from build123d import *

# Parameters (mm, degrees)
SKETCH_3_W          = 11
SKETCH_3_H          = 20
SKETCH_3_R          = 1.6
SKETCH_3_R_2        = 1.225
EXTRUDE_1_DEPTH     = 21.25
SKETCH_4_W          = 3
SKETCH_4_H          = 5.7
CUT_EXTRUDE_1_DEPTH = 7.1


with BuildPart() as part:
    # 草图3 → 凸台-拉伸1 (new body)
    with BuildSketch(Plane.XY):
        with Locations((5.5, 10)):
            Rectangle(SKETCH_3_W, SKETCH_3_H)
        with Locations((3.5, 14.85)):
            Circle(SKETCH_3_R, mode=Mode.SUBTRACT)
        with Locations((3.5, 5.15)):
            Circle(SKETCH_3_R, mode=Mode.SUBTRACT)
        with Locations((8.15, 14.85)):
            Circle(SKETCH_3_R_2, mode=Mode.SUBTRACT)
        with Locations((8.15, 5.15)):
            Circle(SKETCH_3_R_2, mode=Mode.SUBTRACT)
    extrude(amount=EXTRUDE_1_DEPTH)

    # 草图4 → 切除-拉伸1 (cut)
    with BuildSketch(Plane.ZY):
        with Locations((4.5, 14.85)):
            Rectangle(SKETCH_4_W, SKETCH_4_H)
        with Locations((4.5, 5.15)):
            Rectangle(SKETCH_4_W, SKETCH_4_H)
    extrude(amount=-CUT_EXTRUDE_1_DEPTH, mode=Mode.SUBTRACT)


solid = part.part
The model under review builds one solid part; all positions refer to its coordinate system, in mm. A direction names the side the tool comes from. Round coordinates to 2 decimals unless told otherwise and drop trailing zeros. Write each loop counter-clockwise with the first axis right and the second up, starting at its lowest first coordinate (ties: lowest second). Pieces come first, ordered by that corner, then holes. Notation, with made-up numbers: M 79,0.5 L 103,0.5 A11 cw 103,5.5 Z; hole C 12,63 d6. An arc over 180 degrees is marked long. Use a Markdown table: item, result. Add a question column.
Q1. We need section B-B, the plane y = 5.15. State the section outline as (x, z) points (3 decimals), plus the area to 3 significant figures.
Q2. To check wall thickness, follow line 1 (X direction, y = 14.85, z = 18.25) (3 decimals); line 2 (Y direction, x = 3.5, z = 18); line 3 (Y direction, x = 8.25, z = 3.25). State the ranges of each line that lie inside material, in increasing order.
Q3. Insertion check: pin 1 (2.5 mm diameter, centred on x = 3.5, y = 5.15, fed in from +Z); pin 2 (1.1 mm diameter, centred on y = 3.5, z = 5, fed in from -X). Each pin has a flat end and moves straight along its axis. Give the tip position at first contact, or say it passes through.
Q4. Machinability: for faces 4 (the face through (3.292, 6.736, 1.479)), 5 (the face through (4, 17.7, 4)), which of the approach directions +Z, -Z, +X, -X, +Y, -Y give a long, thin tool a straight path to every point of the face, cutting with its end or side? Answer none if there is none.
Q5. We need section A-A, the plane x = 3.5. State the section outline as (y, z) points.
Q6. We need section D-D, the plane z = 13.5. State the section outline as (x, y) points (3 decimals).
Q7. The part is to be moulded in two halves that separate along Y. For faces 1 (the face through (4, 12, 4)), 2 (the face through (5, 0, 10)), 3 (the face through (11, 10, 10)), say which applies: pulls with the +Y half, pulls with the -Y half, needs draft (parallel to the pull), parting line crosses it, or undercut.
Q8. We need section C-C, the plane x = 6. State the section outline as (y, z) points, plus the area to 3 significant figures.
Findings below:
| question | item | result |
|---|---|---|
| 1 | outline | M 0,0 L 1.9,0 L 1.9,3 L 0,3 Z; M 0,6 L 1.9,6 L 1.9,21.25 L 0,21.25 Z; M 5.1,0 L 6.925,0 L 6.925,3 L 5.1,3 Z; M 5.1,6 L 6.925,6 L 6.925,21.25 L 5.1,21.25 Z; M 9.375,0 L 11,0 L 11,21.25 L 9.375,21.25 Z |
| 1 | area | 103 mm² |
| 2 | line 1 | x = 0 to 1.9, 5.1 to 6.925, 9.375 to 11 |
| 2 | line 2 | y = 0 to 3.55, 6.75 to 13.25, 16.45 to 20 |
| 2 | line 3 | y = 0 to 3.93, 6.37 to 13.63, 16.07 to 20 |
| 3 | pin 1 | passes through |
| 3 | pin 2 | stops at x = 7.1 |
| 4 | face 4 | +Z, -Z |
| 4 | face 5 | -X |
| 5 | outline | M 0,0 L 3.55,0 L 3.55,3 L 2.3,3 L 2.3,6 L 3.55,6 L 3.55,21.25 L 0,21.25 Z; M 6.75,0 L 13.25,0 L 13.25,3 L 12,3 L 12,6 L 13.25,6 L 13.25,21.25 L 6.75,21.25 L 6.75,6 L 8,6 L 8,3 L 6.75,3 Z; M 16.45,0 L 20,0 L 20,21.25 L 16.45,21.25 L 16.45,6 L 17.7,6 L 17.7,3 L 16.45,3 Z |
| 6 | outline | M 0,0 L 11,0 L 11,20 L 0,20 Z; hole C 3.5,5.15 d3.2; hole C 3.5,14.85 d3.2; hole C 8.15,5.15 d2.45; hole C 8.15,14.85 d2.45 |
| 7 | face 1 | undercut |
| 7 | face 2 | pulls with the -Y half |
| 7 | face 3 | needs draft |
| 8 | outline | M 0,0 L 20,0 L 20,21.25 L 0,21.25 Z; hole M 2.3,3 L 8,3 L 8,6 L 2.3,6 Z; hole M 12,3 L 17.7,3 L 17.7,6 L 12,6 Z |
| 8 | area | 391 mm² |
